For this review, take the finished solid that the model builds, in its own axes (mm). A direction names the side the tool comes from. Coordinates: 2 decimals unless noted, no trailing zeros. Loops run counter-clockwise (first coordinate to the right, second up) from the corner with the lowest first, then second, coordinate; pieces in that order, holes last. Notation, with made-up numbers: (49, 70.25) - (88, 70.25) arc R30 cw to (88, 107.25) - close; hole circle Ø2 at (86, 64). An arc over 180 degrees is marked (long way). One line per item, written item: value. Start each with the question number.
1. Insertion check: pin 1 (7.5 mm diameter, centred on x = -5, z = 2, fed in from +Y); pin 2 (1 mm diameter, centred on y = 10, z = 13.5, fed in from +X); pin 3 (4 mm diameter, centred on x = -7.25, z = -7.25, fed in from -Y); pin 4 (13 mm diameter, centred on x = 0, z = 0, fed in from -Y). Each pin has a flat end and moves straight along its axis. Give the tip position at first contact, or say it passes through.
2. The part is to be moulded in two halves that separate along X. For faces 3 (the face through (-5.817, -2.465, 6.797)), 4 (the face through (8, 26, 11)), 5 (the face through (31, 10.72, -9.76)), say which applies: released by +X, released by -X, zero draft, split by the parting line, or undercut.
3. Take a section at C-C, the plane y = 7. State the section outline as (x, z) points.
4. Take a section at B-B, the plane x = 0. State the section outline as (y, z) points, and give its area (3 significant figures).
5. For faces 1 (the face through (-1.73, -2.46, 7.81)), 2 (the face through (-0.2, 0, 8.2)), list the 3-axis set-ups (+Z, -Z, +X, -X, +Y, -Y) from which the entire face can be reached by the end or side of a thin tool; tool diameter is ignored.
6. To check wall thickness, follow line 1 (Z direction, x = 0, y = 12); line 2 (Z direction, x = 7, y = 19.5). State the ranges of each line that lie inside material, in increasing order. Write a range as from..to.
7. Take a section at A-A, the plane z = 0. State the section outline as (x, y) points, and give its area (3 significant figures).
8. Take a section at D-D, the plane x = -7. State the section outline as (y, z) points, and give its area (3 significant figures).
```python
from build123d import *

# Parameters (mm, degrees)
SKETCH1_R               = 32.5
SKETCH1_R_2             = 27.5
BOSS_EXTRUDE2_DEPTH     = 26
SKETCH1_R_3             = 17.5
SKETCH1_R_4             = 12.5
BOSS_EXTRUDE2_2_DEPTH   = 26
SKETCH2_R               = 32.5
SKETCH2_R_2             = 8
BOSS_EXTRUDE3_DEPTH     = 5
SKETCH3_R               = 1.5
CUT_EXTRUDE1_DEPTH      = 3
CUT_EXTRUDE1_DEPTH_BACK = 6


with BuildPart() as part:
    # Sketch1 → Boss-Extrude2 (new body)
    with BuildSketch(Plane(origin=(0, 0, 0), x_dir=(1, 0, 0), z_dir=(0, 1, 0))):
        Circle(SKETCH1_R)
        Circle(SKETCH1_R_2, mode=Mode.SUBTRACT)
    extrude(amount=BOSS_EXTRUDE2_DEPTH)



with BuildPart() as body_2:
    # Sketch1 → Boss-Extrude2 2 (new body)
    with BuildSketch(Plane(origin=(0, 0, 0), x_dir=(1, 0, 0), z_dir=(0, 1, 0))):
        Circle(SKETCH1_R_3)
        Circle(SKETCH1_R_4, mode=Mode.SUBTRACT)
    extrude(amount=BOSS_EXTRUDE2_2_DEPTH)


with BuildPart() as part_1:
    add(part.part)

    add(body_2.part)  # Boss-Extrude3 merges body 2
    # Sketch2 → Boss-Extrude3 (add)
    with BuildSketch(Plane(origin=(0, 0, 0), x_dir=(1, 0, 0), z_dir=(0, 1, 0))):
        Circle(SKETCH2_R)
        Circle(SKETCH2_R_2, mode=Mode.SUBTRACT)
    extrude(amount=-BOSS_EXTRUDE3_DEPTH)

    # Sketch3 → Cut-Extrude1 (cut, two sides)
    with BuildSketch(Plane(origin=(0, 0, 0), x_dir=(1, 0, 0), z_dir=(0, 1, 0))) as cut_extrude1_sk:
        with Locations((-7.247844507, 7.247844507)):
            Circle(SKETCH3_R)
        with Locations((7.247844507, 7.247844507)):
            Circle(SKETCH3_R)
        with Locations((7.247844507, -7.247844507)):
            Circle(SKETCH3_R)
        with Locations((-7.247844507, -7.247844507)):
            Circle(SKETCH3_R)
    extrude(amount=CUT_EXTRUDE1_DEPTH, mode=Mode.SUBTRACT)
    extrude(cut_extrude1_sk.sketch, amount=-CUT_EXTRUDE1_DEPTH_BACK, mode=Mode.SUBTRACT)


solid = part_1.part
```
Solutions:
1. pin 1: y = 0
1. pin 2: x = 29.79
1. pin 3: y = -5
1. pin 4: through
2. face 3: undercut
2. face 4: zero draft
2. face 5: split by the parting line
3. outline: circle Ø65 at (0, 0); circle Ø35 at (0, 0); hole circle Ø55 at (0, 0); hole circle Ø25 at (0, 0)
4. outline: (-5, -32.5) - (26, -32.5) - (26, -27.5) - (0, -27.5) - (0, -17.5) - (26, -17.5) - (26, -12.5) - (0, -12.5) - (0, -8) - (-5, -8) - close; (-5, 8) - (0, 8) - (0, 12.5) - (26, 12.5) - (26, 17.5) - (0, 17.5) - (0, 27.5) - (26, 27.5) - (26, 32.5) - (-5, 32.5) - close
4. area: 765 mm2
5. face 1: +Y, -Y
5. face 2: +Y
6. line 1: -32.5..-27.5, -17.5..-12.5, 12.5..17.5, 27.5..32.5
6. line 2: -31.74..-26.59, -16.04..-10.36, 10.36..16.04, 26.59..31.74
7. outline: (-32.5, -5) - (-8, -5) - (-8, 0) - (-12.5, 0) - (-12.5, 26) - (-17.5, 26) - (-17.5, 0) - (-27.5, 0) - (-27.5, 26) - (-32.5, 26) - close; (8, -5) - (32.5, -5) - (32.5, 26) - (27.5, 26) - (27.5, 0) - (17.5, 0) - (17.5, 26) - (12.5, 26) - (12.5, 0) - (8, 0) - close
7. area: 765 mm2
8. outline: (-5, -31.74) - (26, -31.74) - (26, -26.59) - (0, -26.59) - (0, -16.04) - (26, -16.04) - (26, -10.36) - (0, -10.36) - (0, -8.73) - (-5, -8.73) - close; (-5, -5.77) - (0, -5.77) - (0, -3.87) - (-5, -3.87) - close; (-5, 3.87) - (0, 3.87) - (0, 5.77) - (-5, 5.77) - close; (-5, 8.73) - (0, 8.73) - (0, 10.36) - (26, 10.36) - (26, 16.04) - (0, 16.04) - (0, 26.59) - (26, 26.59) - (26, 31.74) - (-5, 31.74) - close
8. area: 812 mm2
